```python
from build123d import *

# Parameters (mm, degrees)
BOSS_EXTRUDE1_DEPTH = 30


with BuildPart() as part:
    # Sketch1 → Boss-Extrude1 (new body)
    with BuildSketch(Plane.XY):
        with BuildLine():
            Line((0, 19), (0, 0))
            Line((0, 0), (1.5, 0))
            Line((1.5, 0), (1.5, 18.5))
            Line((1.5, 18.5), (20, 18.5))
            Line((20, 18.5), (20, 20))
            Line((20, 20), (1, 20))
            ThreePointArc((1, 20), (0.292893219, 19.707106781), (0, 19))
        make_face()
        with BuildLine():
            Line((-1.5, 0), (0, 0))
            Line((0, 0), (0, 19))
            ThreePointArc((0, 19), (0.292893219, 19.707106781), (1, 20))
            Line((1, 20), (20, 20))
            Line((20, 20), (20, 21.5))
            Line((20, 21.5), (1, 21.5))
            ThreePointArc((1, 21.5), (-0.767766953, 20.767766953), (-1.5, 19))
            Line((-1.5, 19), (-1.5, 0))
        make_face()
    extrude(amount=BOSS_EXTRUDE1_DEPTH)


solid = part.part
```
Input: part model. Units: mm. Frame: model coordinates. A direction names the side the tool comes from. Give positions to 0.01 mm unless a question says otherwise; leave off trailing zeros. Order: outer loops, then holes, each group sorted by start corner. A loop starts at its lowest first (then second) coordinate and runs counter-clockwise, first axis right, second up. Notation, with made-up numbers: M 29,73 L 38,73 A26 cw 38,92 Z; hole C 28.25,-31.75 d5. An arc over 180 degrees is marked long. Return JSON: item names as keys, results as strings.
1) Section query A-A on z = 26.75. Output: boundary loops of the cut face in (x, y).
Taken from the geometry:
{"outline": "M -1.5,0 L 1.5,0 L 1.5,18.5 L 20,18.5 L 20,21.5 L 1,21.5 A2.5 ccw -1.5,19 Z"}
2) Line query: L1, parallel to X at y = 17.75, z = 11; L2, parallel to Y at x = 11.25, z = 5; L3, parallel to Y at x = 0.25, z = 20. Output: solid intervals per line, ascending. Write a range as [from, to].
Taken from the geometry:
{"L1": "x = [-1.5, 1.5]", "L2": "y = [18.5, 21.5]", "L3": "y = [0, 21.38]"}
3) Section query C-C on x = 17. Output: boundary loops of the cut face in (y, z).
Taken from the geometry:
{"outline": "M 18.5,0 L 21.5,0 L 21.5,30 L 18.5,30 Z"}
4) Contact query for flat-ended pins moving along their axis: pin 1 (5.5 mm diameter, centred on x = 14, z = 9.5, fed in from -Y); pin 2 (9 mm diameter, centred on y = 9.5, z = 15.5, fed in from +X). Output: stop coordinate, or through.
Taken from the geometry:
{"pin 1": "stops at y = 18.5", "pin 2": "stops at x = 1.5"}
5) Access query for faces 1 (the face through (-1.5, 10, 15)), 2 (the face through (1.5, 9, 15)). Directions: +Z, -Z, +X, -X, +Y, -Y. A direction counts if a zero-diameter tool reaches every point of the face in a straight line with its end or side. Return the directions, or none.
Taken from the geometry:
{"face 1": "+Z, -Z, -X, +Y, -Y", "face 2": "+Z, -Z, +X, -Y"}
6) Section query B-B on y = 6.5. Output: boundary loops of the cut face in (x, z).
Taken from the geometry:
{"outline": "M -1.5,0 L 1.5,0 L 1.5,30 L -1.5,30 Z"}
